The model under review builds one solid part; all positions refer to its coordinate system, in mm. A direction names the side the tool comes from. Round coordinates to 2 decimals unless told otherwise and drop trailing zeros. Write each loop counter-clockwise with the first axis right and the second up, starting at its lowest first coordinate (ties: lowest second). Pieces come first, ordered by that corner, then holes. Notation, with made-up numbers: (70, 14) - (128, 14) arc R17 ccw to (128, 28) - close; hole circle Ø5 at (75, 42.5). An arc over 180 degrees is marked (long way). Write each question's results on one line, items separated by ' | '.
```python
from build123d import *

# Parameters (mm, degrees)
SKETCH1_R          = 9.525
SKETCH1_R_2        = 3.937
EXTRUDE1_DEPTH     = 63.5
CUT_EXTRUDE1_DEPTH = 25.4
CUT_EXTRUDE2_DEPTH = 25.4
SKETCH4_R          = 2.413
SKETCH4_R_2        = 1.8923
CUT_EXTRUDE3_DEPTH = 6.35
CHAMFER2_SIZE      = 2.54
SKETCH5_R          = 12.7
CUT_EXTRUDE4_DEPTH = 67.79886128


with BuildPart() as part:
    # Sketch1 → Extrude1 (new body)
    with BuildSketch(Plane.XY):
        Circle(SKETCH1_R)
        Circle(SKETCH1_R_2, mode=Mode.SUBTRACT)
    extrude(amount=-EXTRUDE1_DEPTH)

    # Sketch2 → Cut-Extrude1 (cut)
    with BuildSketch(Plane.XY):
        with BuildLine():
            Line((-9.525, -3.2004), (9.525, -3.2004))
            Line((9.525, -3.2004), (9.525, 3.2004))
            ThreePointArc((9.525, 3.2004), (0, 10.329891018), (-9.525, 3.2004))
            Line((-9.525, 3.2004), (-9.525, -3.2004))
        make_face()
    extrude(amount=-CUT_EXTRUDE1_DEPTH, mode=Mode.SUBTRACT)

    # Sketch3 → Cut-Extrude2 (cut)
    with BuildSketch(Plane.XY):
        Polygon((0, -9.525), (6.594230769, -9.525), (6.594230769, -8.89), (-6.187179487, -8.89), (-6.187179487, -9.525), align=None)
    extrude(amount=-CUT_EXTRUDE2_DEPTH, mode=Mode.SUBTRACT)

    # Sketch4 → Cut-Extrude3 (cut, symmetric)
    with BuildSketch(Plane.XZ.offset(8.89)):
        with Locations(Location((0, -6.096, 0), (0, 0, 198.152695479))):
            Circle(SKETCH4_R)
        with Locations(Location((0, -18.796, 0), (0, 0, 198.152695479))):
            Circle(SKETCH4_R)
        with Locations(Location((0, -38.995512821, 0), (0, 0, 270))):
            Circle(SKETCH4_R_2)
        with Locations(Location((0, -51.695512821, 0), (0, 0, 270))):
            Circle(SKETCH4_R_2)
    extrude(amount=CUT_EXTRUDE3_DEPTH, both=True, mode=Mode.SUBTRACT)

    # Chamfer2
    chamfer2_edges = [part.edges().sort_by_distance(p)[0] for p in [
        (-9.525, 0, -63.5),
    ]]
    chamfer(chamfer2_edges, length=CHAMFER2_SIZE)

    # Sketch5 → Cut-Extrude4 (cut, through all)
    with BuildSketch(Plane.XZ.offset(8.89)):
        with Locations((0, 11.1125)):
            Circle(SKETCH5_R)
    extrude(amount=-CUT_EXTRUDE4_DEPTH, mode=Mode.SUBTRACT)


solid = part.part
```
Q1. We need section A-A (x = 0). State the section outline as (y, z) points (1 decimal), plus the area to 3 significant figures.
Evaluation:
outline: (-9.5, -61) - (-7, -63.5) - (-3.9, -63.5) - (-3.9, -53.6) - (-9.5, -53.6) - close; (-9.5, -49.8) - (-3.9, -49.8) - (-3.9, -40.9) - (-9.5, -40.9) - close; (-9.5, -37.1) - (-3.9, -37.1) - (-3.9, -21.2) - (-8.9, -21.2) - (-8.9, -25.4) - (-9.5, -25.4) - close; (-8.9, -16.4) - (-3.9, -16.4) - (-3.9, -8.5) - (-8.9, -8.5) - close; (-8.9, -3.7) - (-3.9, -3.7) - (-3.9, -1.6) - (-8.9, -1.6) - close; (3.9, -63.5) - (7, -63.5) - (9.5, -61) - (9.5, -25.4) - (3.9, -25.4) - close | area: 447 mm^2
Q2. We need section B-B (y = 0). State the section outline as (x, z) points (3 decimals), plus the area to 3 significant figures.
Evaluation:
outline: (-9.525, -60.96) - (-6.985, -63.5) - (-3.937, -63.5) - (-3.937, -25.4) - (-9.525, -25.4) - close; (3.937, -63.5) - (6.985, -63.5) - (9.525, -60.96) - (9.525, -25.4) - (3.937, -25.4) - close | area: 419 mm^2
Q3. Insertion check: P1, Ø7.5, axis at x = 1, z = -15, coming from the -Y side; P2, Ø4, axis at x = -1.5, y = 3.5, coming from the +Z side; P3, Ø1, axis at y = 0.5, z = -50, coming from the +X side (3 decimals); P4, Ø3, axis at x = -2, z = -8.5, coming from the +Y side. Each pin has a flat end and moves straight along its axis. Give the tip position at first contact, or say it passes through.
Evaluation:
P1: stops at y = -8.89 | P2: stops at z = -25.4 | P3: stops at x = 9.525 | P4: stops at y = -3.2
Q4. We need section D-D (z = -36). State the section outline as (x, y) points (3 decimals), plus the area to 3 significant figures.
Evaluation:
outline: circle Ø19.05 at (0, 0); hole circle Ø7.874 at (0, 0) | area: 236 mm^2
Q5. For probe 1 along Z at (x, y) = (0, -6.6); probe 2 along X at (y, z) = (0, -32.5) (3 decimals), list the stretches that pass through material, from the lowest coordinate up.
Evaluation:
probe 1: z = -63.5 to -53.59, -49.8 to -40.89, -37.1 to -21.21, -16.38 to -8.51, -3.68 to -1.59 | probe 2: x = -9.525 to -3.937, 3.937 to 9.525
Q6. Tool access review of faces 1 (the cylindrical face through (-0.09, -6.085, -1.587)), 2 (the cylindrical face through (0.083, -6.534, -49.805)), 3 (the conical face through (-0.925, 7.048, -63.377)), 4 (the flat face through (0, -8.89, -13)), 5 (the flat face through (6, -3.2, -13)): name each direction out of +Z, -Z, +X, -X, +Y, -Y from which nothing blocks a thin tool from reaching the whole face with its end or side.
Evaluation:
face 1: +Z, +Y, -Y | face 2: -Y | face 3: -Z | face 4: +Z, +X, -X, -Y | face 5: +Z, +X, -X, +Y
Q7. We need section C-C (z = -11). State the section outline as (x, y) points (3 decimals).
Evaluation:
outline: (-8.971, -3.2) arc R9.525 ccw to (-3.42, -8.89) - (3.42, -8.89) arc R9.525 ccw to (8.971, -3.2) - (2.293, -3.2) arc R3.937 cw to (-2.293, -3.2) - close
Q8. The part is to be moulded in two halves that separate along Z. For faces 6 (the cylindrical face through (-0.034, -3.937, -12.368)), 7 (the cylindrical face through (-2.406, -6.085, -18.612)), 8 (the flat face through (7, -5, 0)), say which applies: released by +Z, released by -Z, zero draft, split by the parting line, or undercut.
Evaluation:
face 6: zero draft | face 7: undercut | face 8: released by +Z
